Verification items for the finished model (mm, model axes). Round coordinates to 2 decimals unless told otherwise and drop trailing zeros. Order: outer loops, then holes, each group sorted by start corner. A loop starts at its lowest first (then second) coordinate and runs counter-clockwise, first axis right, second up. Notation, with made-up numbers: M 69.25,81 L 106.25,81 A15 ccw 106.25,105 Z; hole C -29,-38 d2. An arc over 180 degrees is marked long. Return JSON: item names as keys, results as strings. Group by question number.
Autodesk Inventor part; units mm, degrees
ref_plane "YZ Plane" through (0, 0, 0) normal (1, 0, 0) x (0, 1, 0)
ref_plane "XZ Plane" through (0, 0, 0) normal (0, 1, 0) x (-1, 0, 0)
ref_plane "XY Plane" through (0, 0, 0) normal (0, 0, 1) x (1, 0, 0)
sketch "Sketch1" plane through (0, 0, 0) normal (0, 1, 0) x (-1, 0, 0)
  line L0 (-107.95, 101.6) -> (107.95, 101.6)
  line L1 (107.95, 101.6) -> (107.95, -101.6) construction
  line L2 (107.95, -101.6) -> (-107.95, -101.6)
  line L3 (-107.95, -101.6) -> (-107.95, 101.6)
  line L4 (-107.95, 101.6) -> (107.95, -101.6) construction
  line L5 (107.95, 101.6) -> (-107.95, -101.6) construction
  circle A0 centre (-65.9765, 70.739) radius 28.575 construction
  line L6 (107.95, 101.6) -> (171.45, 101.6)
  line L7 (171.45, 101.6) -> (171.45, -101.6)
  line L8 (171.45, -101.6) -> (107.95, -101.6)
  line L9 (107.95, -101.6) -> (107.95, 101.6) construction
  circle A1 centre (131.7625, 70.739) radius 28.575 construction
  circle A2 centre (139.7, -44.4992) radius 30.1625 construction
  circle A3 centre (32.8287, 67.1746) radius 75.057 construction
  arc A4 (-42.5309, -101.6) -> (105.9516, 44.4492) centre (-65.9765, 70.739) ccw construction
  line L10 (139.7, -25.9224) -> (139.7, -58.8783) construction
  line L11 (157.6605, -26.5386) -> (139.7, -44.4992) construction
  point P0 (0, 0)
  point P1 (121.7395, -26.5386)
  point P2 (121.7395, -62.4597)
  point P3 (157.6605, -62.4597)
  dimension "d0" = 203.2
  dimension "d1" = 215.9
  dimension "d5" = 57.15
  dimension "d9" = 57.15
  dimension "d10" = 197.739
  dimension "d12" = 115.5112
  dimension "d13" = 60.325
  dimension "d14" = 150.114
  dimension "d15" = 172.339
  dimension "d17" = 173.9265
  dimension "d18" = 173.9265
  dimension "d28" = 25.4
  dimension "d31" = 360
  dimension "d33" = 45
  dimension "d79" = 279.4
extrude "Plate1" add sketch "Sketch1" along normal blind 4.7625
hole "Hole1" at (65.9765, 0, 70.739) at (-131.7625, 0, 70.739) direction (0, 1, 0) diameter 28.575 depth 4.7625 tip angle 118
sketch "Sketch2" plane through (0, 0, 0) normal (0, -1, 0) x (1, 0, 0)
  circle A0 centre (65.9765, 70.739) radius 14.2875
  point P0 (0, 0)
  point P1 (-73.7235, -62.611)
  point P2 (-32.4485, -91.186)
  point P3 (-99.1235, -14.986)
  dimension "d41" = 165.1
  dimension "d42" = 85.725
  dimension "d43" = 161.925
  dimension "d44" = 98.425
  dimension "d45" = 139.7
  dimension "d46" = 133.35
hole "Hole3" at (-32.4485, 0, -91.186) at (-73.7235, 0, -62.611) at (-99.1235, 0, -14.986) direction (0, 1, 0) diameter 4.9784 depth 4.7625 tip angle 118
sketch "Sketch3" plane through (0, 0, 0) normal (0, -1, 0) x (1, 0, 0)
  line L0 (107.95, -101.6) -> (-171.45, -101.6)
  line L1 (107.95, 101.6) -> (107.95, -101.6)
  point P0 (0, 0)
  point P1 (95.25, -76.2)
  point P2 (95.25, -25.4)
  dimension "d54" = 50.8
  dimension "d55" = 25.4
  dimension "d56" = 12.7
hole "Hole4" at (95.25, 0, -76.2) at (95.25, 0, -25.4) direction (0, 1, 0) diameter 4.9784 depth 4.7625 tip angle 118
sketch "Sketch4" plane through (0, 0, 0) normal (0, -1, 0) x (1, 0, 0)
  line L0 (-171.45, -101.6) -> (-171.45, 101.6)
  line L1 (107.95, -101.6) -> (-171.45, -101.6)
  line L2 (107.95, 101.6) -> (107.95, -101.6)
  point P0 (0, 0)
  point P1 (-82.55, -95.25)
  point P2 (-69.85, -95.25)
  point P3 (-57.15, -95.25)
  point P4 (63.5, -95.25)
  point P5 (50.8, -95.25)
  point P6 (76.2, -95.25)
  point P7 (-158.75, -95.25)
  dimension "d64" = 12.7
  dimension "d65" = 12.7
  dimension "d66" = 88.9
  dimension "d67" = 6.35
  dimension "d68" = 6.35
  dimension "d69" = 12.7
  dimension "d70" = 12.7
  dimension "d71" = 31.75
  dimension "d141" = 12.7
hole "Hole5" at (-82.55, 0, -95.25) at (-69.85, 0, -95.25) at (-57.15, 0, -95.25) at (63.5, 0, -95.25) at (50.8, 0, -95.25) at (76.2, 0, -95.25) at (-158.75, 0, -95.25) direction (0, 1, 0) diameter 4.9784 depth 4.7625 tip angle 118
fillet "Corner Round1" radius 6.35 4 edges at (-171.45, 2.3813, -101.6) (-171.45, 2.3813, 101.6) (107.95, 2.3813, -101.6) (107.95, 2.3813, 101.6)
sketch "Sketch5" plane through (0, 4.7625, 0) normal (0, -1, 0) x (1, 0, 0)
  circle A0 centre (-131.7625, 70.739) radius 14.2875
  circle A1 centre (-131.7625, 70.739) radius 28.575
  circle A2 centre (65.9765, 70.739) radius 14.2875
  circle A3 centre (65.9765, 70.739) radius 28.575
  line L0 (-165.1, 101.6) -> (101.6, 101.6)
  line L1 (-171.45, -95.25) -> (-171.45, 95.25)
  line L2 (107.95, 95.25) -> (107.95, -95.25)
  point P0 (0, 0)
  point P1 (-165.1, 95.25)
  point P2 (101.6, 95.25)
  point P3 (-50.8, 95.25)
  point P4 (-38.1, 95.25)
  point P5 (-25.4, 95.25)
  dimension "d81" = 57.15
  dimension "d82" = 57.15
  dimension "d83" = 6.35
  dimension "d84" = 6.35
  dimension "d85" = 6.35
  dimension "d86" = 114.3
  dimension "d87" = 12.7
  dimension "d88" = 12.7
hole "Hole6" at (-165.1, 4.7625, 95.25) at (101.6, 4.7625, 95.25) at (-50.8, 4.7625, 95.25) at (-25.4, 4.7625, 95.25) direction (0, -1, 0) diameter 4.9784 depth 4.7625 tip angle 118
sketch "Sketch6" plane through (0, 0, 0) normal (0, -1, 0) x (1, 0, 0)
  line L0 (-171.45, -95.25) -> (-171.45, 95.25)
  point P0 (0, 0)
  point P1 (-165.1, -6.35)
  point P2 (-165.1, 6.35)
  dimension "d96" = 12.7
  dimension "d97" = 6.35
  dimension "d98" = 6.35
hole "Hole7" at (-165.1, 0, -6.35) at (-165.1, 0, 6.35) direction (0, 1, 0) diameter 4.9784 depth 4.7625 tip angle 118
hole "Hole8" at (-25.4, 4.7625, 95.25) at (-50.8, 4.7625, 95.25) direction (0, -1, 0) diameter 4.9784 end through all countersink diameter 10.668 countersink angle 82
sketch "Sketch9" plane through (0, 0, 0) normal (0, -1, 0) x (1, 0, 0)
  line L0 (101.6, -101.6) -> (-165.1, -101.6)
  line L1 (107.95, 101.6) -> (-50.8, 101.6)
  line L2 (-50.8, 101.6) -> (-50.8, -101.6)
  line L3 (-50.8, -101.6) -> (107.95, -101.6)
  line L4 (107.95, -101.6) -> (107.95, 101.6)
  line L5 (-165.1, 101.6) -> (101.6, 101.6)
  line L6 (107.95, 95.25) -> (107.95, -95.25)
  point P0 (0, 0)
  dimension "d153" = 158.75
extrude "Cut2" cut sketch "Sketch9" against normal blind 4.7625
properties part number "PLATE,KICKER,OUTSIDE" material "Aluminum 6061"
1. Thickness scan on line 1 along X through (y, z) = (1.55, -95.25); line 2 along Z through (x, y) = (-165.1, 1.4); line 3 along Z through (x, y) = (-99.5, 0.75). Record the ranges inside material, lowest first. Write a range as from..to.
2. Draft check along X on faces 1 (the face through (-126.29, 2.41, 57.54)), 2 (the face through (-109, 2, -101.6)), 3 (the face through (-54.099, 2.422, 95.177)). Enter one of: +X half, -X half, draft (parallel to the pull), parting line (faces both ways), or undercut.
3. Cross-section at B-B (x = -158.75). Enter the section's corners in (y, z).
4. Cross-section at A-A (z = 6.35). Enter the section's corners in (x, y), plus the area to 3 significant figures.
Computed:
{
 "1": {"line 1": "x = -171.45..-161.24, -156.26..-85.04, -80.06..-72.34, -67.36..-59.64, -54.66..-50.8", "line 2": "z = -101.6..-8.84, -3.86..3.86, 8.84..92.76, 97.74..101.6", "line 3": "z = -101.6..-17.45, -12.53..101.6"},
 "2": {"face 1": "undercut", "face 2": "draft", "face 3": "+X half"},
 "3": {"outline": "M 0,-101.6 L 4.76,-101.6 L 4.76,-97.74 L 0,-97.74 Z; M 0,-92.76 L 4.76,-92.76 L 4.76,101.6 L 0,101.6 Z"},
 "4": {"outline": "M -171.45,0 L -167.59,0 L -167.59,4.76 L -171.45,4.76 Z; M -162.61,0 L -50.8,0 L -50.8,4.76 L -162.61,4.76 Z", "area": "551 mm²"}
}
